from build123d import *

# Parameters (mm, degrees)
PAD_DEPTH       = 5.5
FILLET_R        = 2
SKETCH001_R     = 1.25
POCKET_DEPTH    = 5.501
POCKET001_DEPTH = 4
SKETCH003_R     = 3
SKETCH003_R_2   = 1.25
PAD001_DEPTH    = 2.4
SKETCH004_R     = 2.25
POCKET002_DEPTH = 1.5
SKETCH005_R     = 6.25
POCKET003_DEPTH = 0.8
PAD012_DEPTH    = 1.5
FILLET004_R     = 1.4


with BuildPart() as part:
    # Sketch → Pad (new body)
    with BuildSketch(Plane.XY.offset(0.8)):
        with BuildLine():
            Line((18.151766, -21.733802), (18.151766, -94.733802))
            ThreePointArc((18.151766, -94.733802), (19.030446, -96.855123), (21.151766, -97.733802))
            Line((21.151766, -97.733802), (149.151766, -97.733802))
            ThreePointArc((149.151766, -97.733802), (151.273086, -96.855123), (152.151766, -94.733802))
            Line((152.151766, -94.733802), (152.151766, -21.733802))
            ThreePointArc((152.151766, -21.733802), (151.273086, -19.612482), (149.151766, -18.733802))
            Line((149.151766, -18.733802), (21.151766, -18.733802))
            ThreePointArc((21.151766, -18.733802), (19.030446, -19.612482), (18.151766, -21.733802))
        make_face()
    extrude(amount=-PAD_DEPTH)

    # Fillet
    fillet_edges = [part.edges().sort_by_distance(p)[0] for p in [
        (85.151766, -97.733802, -4.7),
    ]]
    fillet(fillet_edges, radius=FILLET_R)

    # Sketch001 (on Face4 of Fillet) → Pocket (cut, through all)
    with BuildSketch(Plane.XY.offset(0.8)):
        with Locations((23.556766, -24.019802)):
            Circle(SKETCH001_R)
        with Locations((146.746766, -24.019802)):
            Circle(SKETCH001_R)
        with Locations((146.746766, -92.447802)):
            Circle(SKETCH001_R)
        with Locations((23.556766, -92.447802)):
            Circle(SKETCH001_R)
    extrude(amount=-POCKET_DEPTH, mode=Mode.SUBTRACT)

    # Sketch002 (on Face4 of Pocket) → Pocket001 (cut)
    with BuildSketch(Plane.XY.offset(0.8)):
        with BuildLine():
            Line((19.951766, -21.733802), (19.951766, -94.733802))
            ThreePointArc((19.951766, -94.733802), (20.303238, -95.58233), (21.151766, -95.933802))
            Line((21.151766, -95.933802), (149.151766, -95.933802))
            ThreePointArc((149.151766, -95.933802), (150.000294, -95.58233), (150.351766, -94.733802))
            Line((150.351766, -94.733802), (150.351766, -21.733802))
            ThreePointArc((150.351766, -21.733802), (150.000294, -20.885274), (149.151766, -20.533802))
            Line((149.151766, -20.533802), (21.151766, -20.533802))
            ThreePointArc((21.151766, -20.533802), (20.303238, -20.885274), (19.951766, -21.733802))
        make_face()
    extrude(amount=-POCKET001_DEPTH, mode=Mode.SUBTRACT)

    # Sketch003 (on Face31 of Pocket001) → Pad001 (join)
    with BuildSketch(Plane.XY.offset(-3.2)):
        with Locations((23.556766, -24.019802)):
            Circle(SKETCH003_R)
        with Locations((23.556766, -24.019802)):
            Circle(SKETCH003_R_2, mode=Mode.SUBTRACT)
        with Locations((146.746766, -24.019802)):
            Circle(SKETCH003_R)
        with Locations((146.746766, -24.019802)):
            Circle(SKETCH003_R_2, mode=Mode.SUBTRACT)
        with Locations((146.746766, -92.447802)):
            Circle(SKETCH003_R)
        with Locations((146.746766, -92.447802)):
            Circle(SKETCH003_R_2, mode=Mode.SUBTRACT)
        with Locations((23.556766, -92.447802)):
            Circle(SKETCH003_R)
        with Locations((23.556766, -92.447802)):
            Circle(SKETCH003_R_2, mode=Mode.SUBTRACT)
    extrude(amount=PAD001_DEPTH)

    # Sketch004 (on Face8 of Pad001) → Pocket002 (cut)
    with BuildSketch(Plane(origin=(0, 0, -4.7), x_dir=(1, 0, 0), z_dir=(0, 0, -1))):
        with Locations((23.556766, 92.447802)):
            Circle(SKETCH004_R)
        with Locations((146.746766, 92.447802)):
            Circle(SKETCH004_R)
        with Locations((146.746766, 24.019802)):
            Circle(SKETCH004_R)
        with Locations((23.556766, 24.019802)):
            Circle(SKETCH004_R)
    extrude(amount=-POCKET002_DEPTH, mode=Mode.SUBTRACT)

    # Sketch005 (on Face8 of Pocket002) → Pocket003 (cut)
    with BuildSketch(Plane(origin=(0, 0, -4.7), x_dir=(1, 0, 0), z_dir=(0, 0, -1))):
        with Locations((33.151766, 88.733802)):
            Circle(SKETCH005_R)
        with Locations((137.151766, 88.733802)):
            Circle(SKETCH005_R)
        with Locations((137.151766, 27.733802)):
            Circle(SKETCH005_R)
        with Locations((33.151766, 27.733802)):
            Circle(SKETCH005_R)
    extrude(amount=-POCKET003_DEPTH, mode=Mode.SUBTRACT)

    # Sketch024 (on Face4 of Pocket003) → Pad012 (join)
    with BuildSketch(Plane.XY.offset(0.05)):
        with BuildLine():
            ThreePointArc((152.151766, -21.733802), (151.273086, -19.612482), (149.151766, -18.733802))
            Line((142.736766, -18.733802), (149.151766, -18.733802))
            Line((142.736766, -17.233802), (142.736766, -18.733802))
            Line((142.736766, -17.233802), (149.151766, -17.233802))
            ThreePointArc((153.651766, -21.733802), (152.333746, -18.551822), (149.151766, -17.233802))
            Line((153.651766, -21.733802), (153.651766, -94.733802))
            ThreePointArc((149.151766, -99.233802), (152.333746, -97.915783), (153.651766, -94.733802))
            Line((149.151766, -99.233802), (21.151766, -99.233802))
            ThreePointArc((16.651766, -94.733802), (17.969785, -97.915783), (21.151766, -99.233802))
            Line((16.651766, -94.733802), (16.651766, -21.733802))
            ThreePointArc((21.151766, -17.233802), (17.969785, -18.551822), (16.651766, -21.733802))
            Line((21.151766, -17.233802), (131.736766, -17.233802))
            Line((131.736766, -17.233802), (131.736766, -18.733802))
            Line((21.151766, -18.733802), (131.736766, -18.733802))
            ThreePointArc((21.151766, -18.733802), (19.030446, -19.612482), (18.151766, -21.733802))
            Line((18.151766, -94.733802), (18.151766, -21.733802))
            ThreePointArc((18.151766, -94.733802), (19.030446, -96.855123), (21.151766, -97.733802))
            Line((149.151766, -97.733802), (21.151766, -97.733802))
            ThreePointArc((149.151766, -97.733802), (151.273086, -96.855123), (152.151766, -94.733802))
            Line((152.151766, -21.733802), (152.151766, -94.733802))
        make_face()
    extrude(amount=-PAD012_DEPTH)

    # Fillet004
    fillet004_edges = [part.edges().sort_by_distance(p)[0] for p in [
        (16.651766, -58.233802, -1.45),
    ]]
    fillet(fillet004_edges, radius=FILLET004_R)


solid = part.part
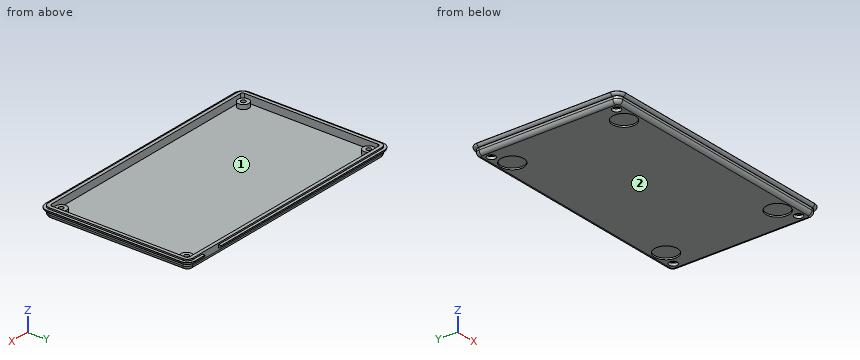
Work out the finished part from the listing and answer in its coordinate system (mm). Face numbers are marked on the shaded views. Round coordinates to 2 decimals unless told otherwise and drop trailing zeros. Write each loop counter-clockwise with the first axis right and the second up, starting at its lowest first coordinate (ties: lowest second). Pieces come first, ordered by that corner, then holes. Notation, with made-up numbers: M 51,37.25 L 94,37.25 A22 ccw 94,45.25 Z; hole C -36.75,86 d1. An arc over 180 degrees is marked long. Use a Markdown table: item, result.
1) The part is cut by section D-D on x = 31. Give the vertices of the cut face in (y, z), plus the area to 3 significant figures.
Taken from the geometry:
| item | result |
|---|---|
| outline | M -99.23,-0.05 A1.4 ccw -97.83,-1.45 L -97.73,-1.45 L -97.73,-2.7 A2 ccw -95.73,-4.7 L -94.6,-4.7 L -94.6,-3.9 L -82.87,-3.9 L -82.87,-4.7 L -33.6,-4.7 L -33.6,-3.9 L -21.87,-3.9 L -21.87,-4.7 L -20.73,-4.7 A2 ccw -18.73,-2.7 L -18.73,-1.45 L -18.63,-1.45 A1.4 ccw -17.23,-0.05 L -17.23,0.05 L -18.73,0.05 L -18.73,0.8 L -20.53,0.8 L -20.53,-3.2 L -95.93,-3.2 L -95.93,0.8 L -97.73,0.8 L -97.73,0.05 L -99.23,0.05 Z |
| area | 116 mm2 |
2) Determine the mould class of the marked faces 1 and 2 for opening direction Y: pulls with the +Y half, pulls with the -Y half, needs draft (parallel to the pull), parting line crosses it, or undercut.
Taken from the geometry:
| item | result |
|---|---|
| face 1 | undercut |
| face 2 | needs draft |
3) Consider line 1 (X direction, y = -28, z = -4.05); line 2 (X direction, y = -31, z = -0.15); line 3 (Y direction, x = 107, z = -2.4). Determine where each line is inside the solid, lowest interval first. Write a range as [from, to].
Taken from the geometry:
| item | result |
|---|---|
| line 1 | x = [18.68, 26.91], [39.4, 130.91], [143.4, 151.63] |
| line 2 | x = [16.66, 19.95], [150.35, 153.65] |
| line 3 | y = [-97.73, -95.93], [-20.53, -18.73] |
4) Flat-ended cylindrical pins translate along their axes: pin 1 (0.8 mm diameter, centred on y = -60.5, z = 0.5, fed in from -X); pin 2 (4 mm diameter, centred on x = 146.75, y = -92.45, fed in from +Z); pin 3 (3.5 mm diameter, centred on x = 33.5, y = -29, fed in from -Z). Find the tip coordinate at first contact, or state that the pin passes through.
Taken from the geometry:
| item | result |
|---|---|
| pin 1 | stops at x = 18.15 |
| pin 2 | stops at z = -0.8 |
| pin 3 | stops at z = -3.9 |
5) The part is cut by section B-B on x = 73. Give the vertices of the cut face in (y, z), plus the area to 3 significant figures.
Taken from the geometry:
| item | result |
|---|---|
| outline | M -99.23,-0.05 A1.4 ccw -97.83,-1.45 L -97.73,-1.45 L -97.73,-2.7 A2 ccw -95.73,-4.7 L -20.73,-4.7 A2 ccw -18.73,-2.7 L -18.73,-1.45 L -18.63,-1.45 A1.4 ccw -17.23,-0.05 L -17.23,0.05 L -18.73,0.05 L -18.73,0.8 L -20.53,0.8 L -20.53,-3.2 L -95.93,-3.2 L -95.93,0.8 L -97.73,0.8 L -97.73,0.05 L -99.23,0.05 Z |
| area | 135 mm2 |
6) The part is cut by section C-C on y = -86. Give the vertices of the cut face in (x, z).
Taken from the geometry:
| item | result |
|---|---|
| outline | M 16.65,-0.05 A1.4 ccw 18.05,-1.45 L 18.15,-1.45 L 18.15,-2.7 A2 ccw 20.15,-4.7 L 27.53,-4.7 L 27.53,-3.9 L 38.77,-3.9 L 38.77,-4.7 L 131.53,-4.7 L 131.53,-3.9 L 142.77,-3.9 L 142.77,-4.7 L 150.15,-4.7 A2 ccw 152.15,-2.7 L 152.15,-1.45 L 152.25,-1.45 A1.4 ccw 153.65,-0.05 L 153.65,0.05 L 152.15,0.05 L 152.15,0.8 L 150.35,0.8 L 150.35,-3.2 L 19.95,-3.2 L 19.95,0.8 L 18.15,0.8 L 18.15,0.05 L 16.65,0.05 Z |
7) The part is cut by section A-A on y = -65.5. Give the vertices of the cut face in (x, z).
Taken from the geometry:
| item | result |
|---|---|
| outline | M 16.65,-0.05 A1.4 ccw 18.05,-1.45 L 18.15,-1.45 L 18.15,-2.7 A2 ccw 20.15,-4.7 L 150.15,-4.7 A2 ccw 152.15,-2.7 L 152.15,-1.45 L 152.25,-1.45 A1.4 ccw 153.65,-0.05 L 153.65,0.05 L 152.15,0.05 L 152.15,0.8 L 150.35,0.8 L 150.35,-3.2 L 19.95,-3.2 L 19.95,0.8 L 18.15,0.8 L 18.15,0.05 L 16.65,0.05 Z |
